Autodesk Inventor part; units mm, degrees
ref_plane "YZ Plane" through (0, 0, 0) normal (1, 0, 0) x (0, 1, 0)
ref_plane "XZ Plane" through (0, 0, 0) normal (0, 1, 0) x (-1, 0, 0)
ref_plane "XY Plane" through (0, 0, 0) normal (0, 0, 1) x (1, 0, 0)
sketch "Sketch2" plane through (0, 0, 0) normal (0, 1, 0) x (-1, 0, 0)
  line L0 (-304.8, 508) -> (304.8, 508)
  line L1 (304.8, 508) -> (304.8, -508)
  line L2 (304.8, -508) -> (-304.8, -508)
  line L3 (-304.8, -508) -> (-304.8, 508)
  line L4 (-304.8, 508) -> (304.8, -508) construction
  line L5 (304.8, 508) -> (-304.8, -508) construction
  point P0 (0, 0)
  dimension "d2" = 609.6
  dimension "d3" = 1016
extrude "Extrusion1" add sketch "Sketch2" along normal blind 609.6
sketch "Sketch3" plane through (304.8, 0, 508) normal (1, 0, 0) x (0, 0, -1)
  line L0 (0, 0) -> (1016, 0)
  line L1 (1016, 0) -> (1016, 609.6)
  line L2 (0, 609.6) -> (1016, 609.6)
  line L3 (0, 0) -> (0, 609.6)
  line L4 (0, 0) -> (0, 609.6)
  line L5 (1016, 0) -> (1016, 609.6)
  line L6 (1016, 0) -> (0, 0)
  line L7 (0, 304.8) -> (1016, 304.8)
  line L8 (1016, 304.8) -> (1016, 0)
  line L9 (1016, 0) -> (0, 0)
  line L10 (0, 0) -> (0, 304.8)
  line L11 (0, 304.8) -> (1016, 304.8)
  line L12 (1016, 304.8) -> (1016, 609.6)
  line L13 (1016, 609.6) -> (0, 609.6)
  line L14 (0, 609.6) -> (0, 304.8)
  line L15 (977.9, 266.7) -> (38.1, 266.7)
  line L16 (38.1, 266.7) -> (38.1, 38.1)
  line L17 (38.1, 38.1) -> (977.9, 38.1)
  line L18 (977.9, 38.1) -> (977.9, 266.7)
  line L19 (977.9, 342.9) -> (38.1, 342.9)
  line L20 (38.1, 342.9) -> (38.1, 571.5)
  line L21 (38.1, 571.5) -> (977.9, 571.5)
  line L22 (977.9, 571.5) -> (977.9, 342.9)
  point P0 (508, 0)
  dimension "d5" = 38.1
  dimension "d6" = 38.1
extrude "Extrusion2" add sketch "Sketch3" along normal blind 25.4 contours L18 L17 L16 L15 | L19 L20 L21 L22
sketch "Sketch4" plane through (304.8, 38.1, 469.9) normal (0, 0, 1) x (1, 0, 0)
  line L0 (0, 304.8) -> (0, 533.4)
  line L1 (0, 304.8) -> (25.4, 304.8)
  line L2 (25.4, 533.4) -> (25.4, 304.8)
  line L3 (0, 533.4) -> (25.4, 533.4)
  line L4 (0, 0) -> (0, 228.6)
  line L5 (0, 0) -> (25.4, 0)
  line L6 (25.4, 228.6) -> (25.4, 0)
  line L7 (0, 228.6) -> (25.4, 228.6)
  line L8 (25.4, 228.6) -> (25.4, 0)
  line L9 (25.4, 228.6) -> (25.4, 254)
  line L10 (0, 228.6) -> (25.4, 228.6)
  line L11 (25.4, 254) -> (0, 228.6)
  line L12 (25.4, 533.4) -> (25.4, 304.8)
  line L13 (25.4, 533.4) -> (25.4, 558.8)
  line L14 (0, 533.4) -> (25.4, 533.4)
  line L15 (25.4, 558.8) -> (0, 533.4)
  point P0 (-304.8, -38.1)
  dimension "d9" = 25.4
  dimension "d10" = 25.4
extrude "Extrusion3" add sketch "Sketch4" against normal up to surface (939.8 mm away) contours L15 L13 L3 | L11 L9 L7
properties part number "drawer"
For this review, take the finished solid that the model builds, in its own axes (mm). A direction names the side the tool comes from. Give positions to 0.01 mm unless a question says otherwise; leave off trailing zeros. One line per item, written item: value.
1) The part is to be moulded in two halves that separate along Y. For faces 5 (the flat face through (4, 0, 7)), 6 (the flat face through (330.2, 167, 7)), 7 (the flat face through (317.7, 279.6, 6.6)), 8 (the flat face through (4, 609.6, 7)), say which applies: +Y half, -Y half, draft (parallel to the pull), parting line (faces both ways), or undercut.
Results are:
face 5: -Y half
face 6: draft
face 7: undercut
face 8: +Y half
2) For line 1 (X direction, y = 310, z = -248); line 2 (X direction, y = 282.5, z = -389.5); line 3 (X direction, y = 279, z = -357), list the stretches that pass through material, from the lowest coordinate up. Write a range as from..to.
Results are:
line 1: x = -304.8..304.8
line 2: x = -304.8..304.8, 320.6..330.2
line 3: x = -304.8..304.8, 317.1..330.2
3) For faces 1 (the flat face through (317, 468, 469.9)), 2 (the flat face through (317, 38.1, 7)), 3 (the flat face through (317, 342.9, -7)), 4 (the flat face through (317, 163, -469.9)), list the 3-axis set-ups (+Z, -Z, +X, -X, +Y, -Y) from which the entire face can be reached by the end or side of a thin tool; tool diameter is ignored.
Results are:
face 1: +Z, +X, +Y, -Y
face 2: +Z, -Z, +X, -Y
face 3: +Z, -Z, +X
face 4: -Z, +X, +Y, -Y
4) For P1, Ø12.5, axis at x = 322, y = 507, coming from the +Z side; P2, Ø7.5, axis at x = 316.5, z = -163.5, coming from the -Y side, all flat-tipped, find the tip position at first contact; note any pin that passes through.
Results are:
P1: stops at z = 469.9
P2: stops at y = 38.1
